from build123d import *

# Parameters (mm, degrees)
F0_R     = 44.5
F0_R_2   = 41
F1_DEPTH = 100
F2_R     = 2
F3_R     = 0.5
F4_DEPTH = 2


with BuildPart() as f1:
    # F0 (on Top) → F1 (new body)
    with BuildSketch(Plane.XY):
        Circle(F0_R)
        Circle(F0_R_2, mode=Mode.SUBTRACT)
    extrude(amount=F1_DEPTH)

    # F2
    f2_edges = [f1.edges().sort_by_distance(p)[0] for p in [
        (-44.5, 0, 100),
        (-44.5, 0, 0),
    ]]
    fillet(f2_edges, radius=F2_R)

    # F3
    f3_edges = [f1.edges().sort_by_distance(p)[0] for p in [
        (-41, 0, 100),
    ]]
    fillet(f3_edges, radius=F3_R)

    # F0 (on Top) → F4 (join)
    with BuildSketch(Plane.XY):
        Circle(F0_R_2)
    extrude(amount=F4_DEPTH)


solid = f1.part
Geometry: final body of the model. Coordinates: model frame, mm. A direction names the side the tool comes from. Give positions to 0.01 mm unless a question says otherwise; leave off trailing zeros. Write each loop counter-clockwise with the first axis right and the second up, starting at its lowest first coordinate (ties: lowest second). Pieces come first, ordered by that corner, then holes. Notation, with made-up numbers: M 77,41 L 133,41 A16 ccw 133,52 Z; hole C -33,-5 d3. An arc over 180 degrees is marked long. Answer in a Markdown table with one row per item. Add a question column.
(1) Ray query, line 1 (Y direction, x = 0, z = 32); line 2 (Z direction, x = -20, y = -22); line 3 (Z direction, x = 33, y = 25). Return the intervals inside material, ascending.
(2) Section C-C on z = 43. Return loops of the section in (x, y), and give its area (3 significant figures).
(3) Section A-A on y = 0. Return loops of the section in (x, z), and give its area (3 significant figures).
(4) Mould query, pull axis Y, two halves, no side actions, for faces 1 (the flat face through (-1, 1, 2)), 2 (the flat face through (-1, 1, 0)), 3 (the cylindrical face through (-32.798, 30.075, 49.328)). Classes: +Y half, -Y half, draft (parallel to the pull), parting line (faces both ways), or undercut.
(5) First-contact query: pin 1 (1.5 mm diameter, centred on x = 7, y = -12, fed in from +Z); pin 2 (8 mm diameter, centred on x = -8.5, z = 76.5, fed in from -Y); pin 3 (6 mm diameter, centred on y = -33.5, z = 75, fed in from -X). Flat tips, straight axial feed; report the tip coordinate or a pass-through.
(6) Reachability of faces 4 (the flat face through (9, -41, 100)), 5 (the cylindrical face through (-9, -40, 50)) from +Z, -Z, +X, -X, +Y, -Y: full face, straight path, thin tool, end or side. Return the list, or none.
Result set:
| question | item | result |
|---|---|---|
| 1 | line 1 | y = -44.5 to -41, 41 to 44.5 |
| 1 | line 2 | z = 0 to 2 |
| 1 | line 3 | z = 0 to 99.99 |
| 2 | outline | C 0,0 d89; hole C 0,0 d82 |
| 2 | area | 940 mm^2 |
| 3 | outline | M -44.5,2 A2 ccw -42.5,0 L 42.5,0 A2 ccw 44.5,2 L 44.5,98 A2 ccw 42.5,100 L 41.5,100 A0.5 ccw 41,99.5 L 41,2 L -41,2 L -41,99.5 A0.5 ccw -41.5,100 L -42.5,100 A2 ccw -44.5,98 Z |
| 3 | area | 860 mm^2 |
| 4 | face 1 | undercut |
| 4 | face 2 | draft |
| 4 | face 3 | parting line |
| 5 | pin 1 | stops at z = 2 |
| 5 | pin 2 | stops at y = -44.27 |
| 5 | pin 3 | stops at x = -32.4 |
| 6 | face 4 | +Z, +X, -X, +Y, -Y |
| 6 | face 5 | +Z |
